Verification items for the finished model (mm, model axes). A direction names the side the tool comes from. Coordinates: 2 decimals unless noted, no trailing zeros. Write each loop counter-clockwise with the first axis right and the second up, starting at its lowest first coordinate (ties: lowest second). Pieces come first, ordered by that corner, then holes.
```python
from build123d import *

# Parameters (mm, degrees)
SKETCH_R        = 1.6
PAD_DEPTH       = 9
SKETCH001_W     = 62.43
SKETCH001_H     = 4.25
POCKET_DEPTH    = 6
POCKET001_DEPTH = 3
FILLET_R        = 4


with BuildPart() as part:
    # Sketch → Pad (new body)
    with BuildSketch(Plane.XY):
        with BuildLine():
            Line((0, 0), (94, 0))
            Line((94, 0), (94, 23.275))
            ThreePointArc((94, 23.275), (93.56066, 24.33566), (92.5, 24.775))
            Line((92.5, 24.775), (84.5, 24.775))
            ThreePointArc((83, 26.275), (83.43934, 25.21434), (84.5, 24.775))
            Line((83, 26.275), (83, 42.425))
            ThreePointArc((84.5, 43.925), (83.43934, 43.48566), (83, 42.425))
            Line((84.5, 43.925), (92.5, 43.925))
            ThreePointArc((92.5, 43.925), (93.56066, 44.36434), (94, 45.425))
            Line((94, 45.425), (94, 68.7))
            Line((94, 68.7), (0, 68.7))
            Line((0, 68.7), (0, 0))
        make_face()
        with Locations((3.45, 65.25)):
            Circle(SKETCH_R, mode=Mode.SUBTRACT)
        with Locations((90.55, 65.25)):
            Circle(SKETCH_R, mode=Mode.SUBTRACT)
        with Locations((90.55, 3.45)):
            Circle(SKETCH_R, mode=Mode.SUBTRACT)
        with Locations((3.45, 3.45)):
            Circle(SKETCH_R, mode=Mode.SUBTRACT)
        with BuildLine():
            ThreePointArc((68.95, 10.65), (70.45, 9.15), (71.95, 10.65))
            Line((71.95, 13.4), (71.95, 10.65))
            Line((74.7, 13.4), (71.95, 13.4))
            ThreePointArc((74.7, 13.4), (76.2, 14.9), (74.7, 16.4))
            Line((71.95, 16.4), (74.7, 16.4))
            Line((71.95, 19.15), (71.95, 16.4))
            ThreePointArc((71.95, 19.15), (70.45, 20.65), (68.95, 19.15))
            Line((68.95, 16.4), (68.95, 19.15))
            Line((66.2, 16.4), (68.95, 16.4))
            ThreePointArc((66.2, 16.4), (64.7, 14.9), (66.2, 13.4))
            Line((68.95, 13.4), (66.2, 13.4))
            Line((68.95, 10.65), (68.95, 13.4))
        make_face(mode=Mode.SUBTRACT)
        with BuildLine():
            ThreePointArc((69, 49.55), (70.45, 48.1), (71.9, 49.55))
            Line((71.9, 52.35), (71.9, 49.55))
            Line((74.7, 52.35), (71.9, 52.35))
            ThreePointArc((74.7, 52.35), (76.15, 53.8), (74.7, 55.25))
            Line((71.9, 55.25), (74.7, 55.25))
            Line((71.9, 58.05), (71.9, 55.25))
            ThreePointArc((71.9, 58.05), (70.45, 59.5), (69, 58.05))
            Line((69, 55.25), (69, 58.05))
            Line((66.2, 55.25), (69, 55.25))
            ThreePointArc((66.2, 55.25), (64.75, 53.8), (66.2, 52.35))
            Line((69, 52.35), (66.2, 52.35))
            Line((69, 49.55), (69, 52.35))
        make_face(mode=Mode.SUBTRACT)
        with BuildLine():
            ThreePointArc((14.05, 30.3), (13, 29.25), (14.05, 28.2))
            Line((14.05, 28.2), (26.25, 28.2))
            ThreePointArc((26.25, 28.2), (27.3, 29.25), (26.25, 30.3))
            Line((14.05, 30.3), (26.25, 30.3))
        make_face(mode=Mode.SUBTRACT)
        with BuildLine():
            ThreePointArc((14.05, 35.4), (13, 34.35), (14.05, 33.3))
            Line((14.05, 33.3), (26.25, 33.3))
            ThreePointArc((26.25, 33.3), (27.3, 34.35), (26.25, 35.4))
            Line((14.05, 35.4), (26.25, 35.4))
        make_face(mode=Mode.SUBTRACT)
        with BuildLine():
            ThreePointArc((15.05, 25.2), (14, 24.15), (15.05, 23.1))
            Line((15.05, 23.1), (26.25, 23.1))
            ThreePointArc((26.25, 23.1), (27.3, 24.15), (26.25, 25.2))
            Line((15.05, 25.2), (26.25, 25.2))
        make_face(mode=Mode.SUBTRACT)
        with BuildLine():
            ThreePointArc((16.15, 20.1), (15.1, 19.05), (16.15, 18))
            Line((16.15, 18), (26.25, 18))
            ThreePointArc((26.25, 18), (27.3, 19.05), (26.25, 20.1))
            Line((16.15, 20.1), (26.25, 20.1))
        make_face(mode=Mode.SUBTRACT)
        with BuildLine():
            ThreePointArc((17.85, 15), (16.8, 13.95), (17.85, 12.9))
            Line((17.85, 12.9), (26.25, 12.9))
            ThreePointArc((26.25, 12.9), (27.3, 13.95), (26.25, 15))
            Line((17.85, 15), (26.25, 15))
        make_face(mode=Mode.SUBTRACT)
        with BuildLine():
            ThreePointArc((14.05, 40.5), (13, 39.45), (14.05, 38.4))
            Line((14.05, 38.4), (26.25, 38.4))
            ThreePointArc((26.25, 38.4), (27.3, 39.45), (26.25, 40.5))
            Line((14.05, 40.5), (26.25, 40.5))
        make_face(mode=Mode.SUBTRACT)
        with BuildLine():
            ThreePointArc((15.05, 45.6), (14, 44.55), (15.05, 43.5))
            Line((15.05, 43.5), (26.25, 43.5))
            ThreePointArc((26.25, 43.5), (27.3, 44.55), (26.25, 45.6))
            Line((15.05, 45.6), (26.25, 45.6))
        make_face(mode=Mode.SUBTRACT)
        with BuildLine():
            ThreePointArc((16.15, 50.7), (15.1, 49.65), (16.15, 48.6))
            Line((16.15, 48.6), (26.25, 48.6))
            ThreePointArc((26.25, 48.6), (27.3, 49.65), (26.25, 50.7))
            Line((16.15, 50.7), (26.25, 50.7))
        make_face(mode=Mode.SUBTRACT)
        with BuildLine():
            ThreePointArc((17.85, 55.8), (16.8, 54.75), (17.85, 53.7))
            Line((17.85, 53.7), (26.25, 53.7))
            ThreePointArc((26.25, 53.7), (27.3, 54.75), (26.25, 55.8))
            Line((17.85, 55.8), (26.25, 55.8))
        make_face(mode=Mode.SUBTRACT)
        with BuildLine():
            ThreePointArc((30.35, 15), (29.3, 13.95), (30.35, 12.9))
            Line((30.35, 12.9), (33.25, 12.9))
            ThreePointArc((33.25, 12.9), (34.3, 13.95), (33.25, 15))
            Line((30.35, 15), (33.25, 15))
        make_face(mode=Mode.SUBTRACT)
    extrude(amount=PAD_DEPTH)

    # Sketch001 (on Face82 of Pad) → Pocket (cut)
    with BuildSketch(Plane.XY.offset(9)):
        with Locations((55.885, 66.575)):
            Rectangle(SKETCH001_W, SKETCH001_H)
        with BuildLine():
            Line((4.5, 60.05), (4.5, 8.1))
            ThreePointArc((4.5, 8.1), (4.792893, 7.392893), (5.5, 7.1))
            Line((5.5, 7.1), (83.5, 7.1))
            ThreePointArc((83.5, 7.1), (84.207107, 7.392893), (84.5, 8.1))
            Line((84.5, 8.1), (84.5, 24.775))
            Line((84.5, 24.775), (84.5, 43.925))
            Line((84.5, 43.925), (88.9, 43.925))
            Line((88.9, 43.925), (88.9, 53.15))
            ThreePointArc((88.9, 53.15), (88.607107, 53.857107), (87.9, 54.15))
            Line((87.9, 54.15), (85.3, 54.15))
            ThreePointArc((84.3, 55.15), (84.592893, 54.442893), (85.3, 54.15))
            Line((84.3, 55.15), (84.3, 60.05))
            ThreePointArc((84.3, 60.05), (84.007107, 60.757107), (83.3, 61.05))
            Line((83.3, 61.05), (5.5, 61.05))
            ThreePointArc((5.5, 61.05), (4.792893, 60.757107), (4.5, 60.05))
        make_face()
    extrude(amount=-POCKET_DEPTH, mode=Mode.SUBTRACT)

    # Sketch002 (on Face4 of Pocket) → Pocket001 (cut)
    with BuildSketch(Plane.XY.offset(9)):
        with BuildLine():
            Line((88.9, 7.29), (88.9, 61.52))
            ThreePointArc((88.9, 61.52), (88.607107, 62.227107), (87.9, 62.52))
            Line((87.9, 62.52), (3.9, 62.52))
            ThreePointArc((3.9, 62.52), (3.192893, 62.227107), (2.9, 61.52))
            Line((2.9, 61.52), (2.9, 7.29))
            ThreePointArc((2.9, 7.29), (3.192893, 6.582893), (3.9, 6.29))
            Line((3.9, 6.29), (87.9, 6.29))
            ThreePointArc((87.9, 6.29), (88.607107, 6.582893), (88.9, 7.29))
        make_face()
    extrude(amount=-POCKET001_DEPTH, mode=Mode.SUBTRACT)

    # Fillet
    fillet_edges = [part.edges().sort_by_distance(p)[0] for p in [
        (94, 68.7, 4.5),
        (94, 0, 4.5),
        (0, 0, 4.5),
        (0, 68.7, 4.5),
    ]]
    fillet(fillet_edges, radius=FILLET_R)


solid = part.part
```
1. Material ranges on L1, parallel to X at y = 49.5, z = 2.25; L2, parallel to Y at x = 16.5, z = 7.75; L3, parallel to Y at x = 3.45, z = 4.25, recorded low to high.
2. Sectioned sample at C-C, the plane z = 8. Give the number of separate pieces and of enclosed holes in the cut face, and give its area (3 significant figures).
3. Tool access check on faces 3 (the flat face through (46, 62.52, 8)), 4 (the flat face through (87.1, 67, 6)), 5 (the flat face through (43, 4, 9)), 6 (the flat face through (68, 16.4, 1)), 7 (the flat face through (94, 55, 4)). Record the directions out of +Z, -Z, +X, -X, +Y, -Y that give a thin tool (end or side, any length) a straight path to the whole face; none if there is none.
4. Sectioned sample at B-B, the plane y = 22. Record the boundary of the cut face in (x, z).
5. Gauge pin test, flat ends, axial feed: P1, Ø1.5, axis at y = 34.5, z = 8, coming from the +X side; P2, Ø5, axis at x = 66, z = 6.5, coming from the +Y side; P3, Ø1.5, axis at x = 50.5, y = 39.5, coming from the +Z side. Record the tip position at first contact, or that the pin passes through.
6. Sectioned sample at D-D, the plane x = 39. Record the boundary of the cut face in (y, z), and give its area (3 significant figures).
7. Sectioned sample at A-A, the plane y = 29.25. Record the boundary of the cut face in (x, z), and give its area (3 significant figures).
8. Draft check along Y on faces 1 (the flat face through (55, 67, 3)), 2 (the flat face through (20, 28.2, 1)). Enter one of: pulls with the +Y half, pulls with the -Y half, needs draft (parallel to the pull), parting line crosses it, or undercut.
Outcome:
1. L1: x = 0 to 15.11, 27.29 to 69, 71.9 to 94
1. L2: y = 0 to 6.29, 62.52 to 68.7
1. L3: y = 0.04 to 1.85, 5.05 to 63.65, 66.85 to 68.66
2. separate pieces: 1
2. enclosed holes: 4
2. area: 1,210 mm2
3. face 3: +Z
3. face 4: +Z, +Y
3. face 5: +Z, +X, -X, +Y, -Y
3. face 6: +Z, -Z
3. face 7: +Z, -Z, +X, +Y, -Y
4. outline: (0, 0) - (94, 0) - (94, 9) - (88.9, 9) - (88.9, 6) - (84.5, 6) - (84.5, 3) - (4.5, 3) - (4.5, 6) - (2.9, 6) - (2.9, 9) - (0, 9) - close
5. P1: stops at x = 2.9
5. P2: stops at y = 64.45
5. P3: stops at z = 3
6. outline: (0, 0) - (68.7, 0) - (68.7, 3) - (64.45, 3) - (64.45, 9) - (62.52, 9) - (62.52, 6) - (61.05, 6) - (61.05, 3) - (7.1, 3) - (7.1, 6) - (6.29, 6) - (6.29, 9) - (0, 9) - close
6. area: 262 mm2
7. outline: (0, 0) - (13, 0) - (13, 3) - (4.5, 3) - (4.5, 6) - (2.9, 6) - (2.9, 9) - (0, 9) - close; (27.3, 0) - (83, 0) - (83, 3) - (27.3, 3) - close
7. area: 228 mm2
8. face 1: needs draft
8. face 2: undercut
